Answer from the drawing. Dimensions are ordinates in mm from the lowest x, y and z of the part. A direction names the side the tool comes from. Round coordinates to 2 decimals unless told otherwise and drop trailing zeros. Loops run counter-clockwise (first coordinate to the right, second up) from the corner with the lowest first, then second, coordinate; pieces in that order, holes last. Notation, with made-up numbers: M -10.75,47 L 22.25,47 A21 ccw 22.25,57 Z; hole C 24.5,5.25 d10. An arc over 180 degrees is marked long. Answer as a JSON object with one key per item and string values.
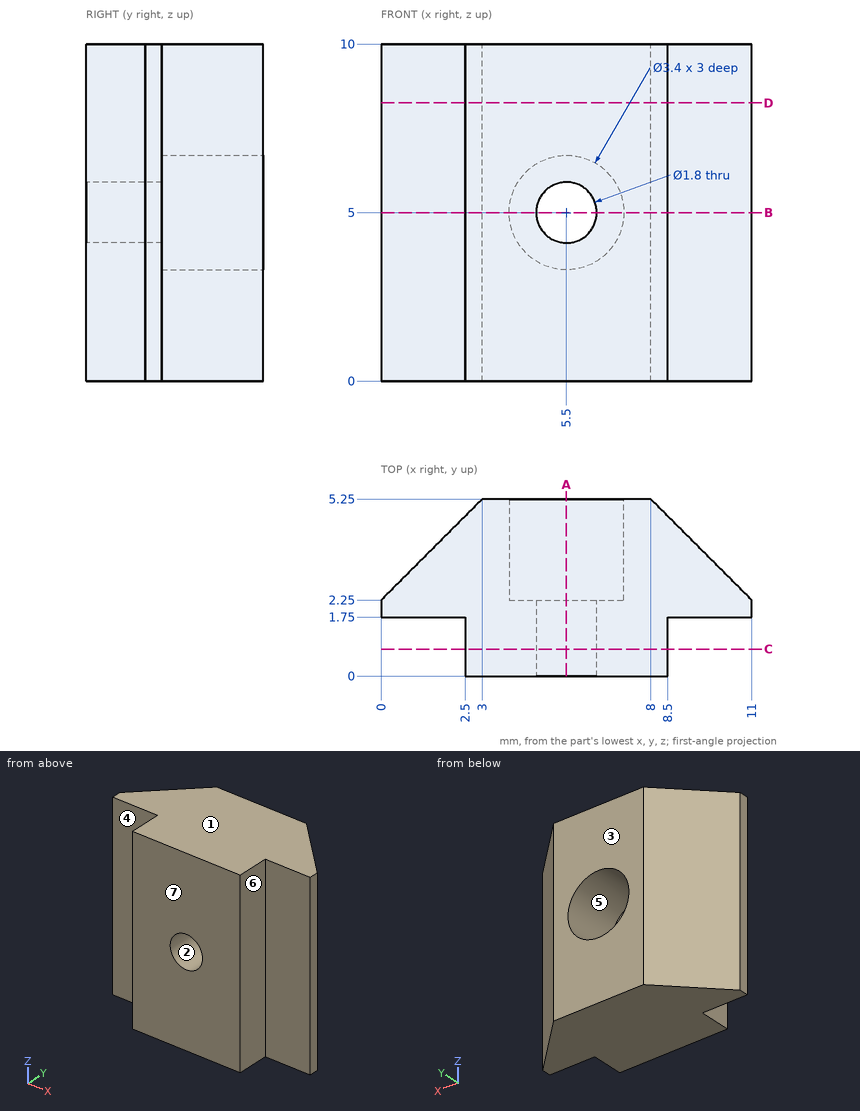
Item 1: The part is cut by section B-B (z = 5). Give the vertices of the cut face in (x, y).
Values follow:
{"outline": "M 0,1.75 L 2.5,1.75 L 2.5,0 L 4.6,0 L 4.6,2.25 L 3.8,2.25 L 3.8,5.25 L 3,5.25 L 0,2.25 Z; M 6.4,0 L 8.5,0 L 8.5,1.75 L 11,1.75 L 11,2.25 L 8,5.25 L 7.2,5.25 L 7.2,2.25 L 6.4,2.25 Z"}
Item 2: Straight lines are drawn through the part: line 1 (Z direction, x = 5.5, y = 0.45); line 2 (X direction, y = 1.6, z = 1); line 3 (X direction, y = 3.6, z = 4.5). For each, find the intervals that lie inside material, in ascending order.
Values follow:
{"line 1": "0 to 4.1, 5.9 to 10", "line 2": "2.5 to 8.5", "line 3": "1.35 to 3.88, 7.12 to 9.65"}
Item 3: Flat-ended cylindrical pins translate along their axes: P1, Ø1.4, axis at y = 0.5, z = 4.5, coming from the -X side; P2, Ø2, axis at x = 10.5, z = 3, coming from the -Y side; P3, Ø1.1, axis at x = 5.5, z = 5, coming from the -Y side; P4, Ø1, axis at y = 3, z = 6, coming from the -X side. Find the tip coordinate at first contact, or state that the pin passes through.
Values follow:
{"P1": "x = 2.5", "P2": "y = 1.75", "P3": "through", "P4": "x = 0.25"}
Item 4: Determine the mould class of the marked faces 1, 2 and 3 for opening direction Z: released by +Z, released by -Z, zero draft, split by the parting line, or undercut.
Values follow:
{"face 1": "released by +Z", "face 2": "undercut", "face 3": "zero draft"}
Item 5: The part is cut by section A-A (x = 5.5). Give the vertices of the cut face in (y, z).
Values follow:
{"outline": "M 0,0 L 5.25,0 L 5.25,3.3 L 2.25,3.3 L 2.25,4.1 L 0,4.1 Z; M 0,5.9 L 2.25,5.9 L 2.25,6.7 L 5.25,6.7 L 5.25,10 L 0,10 Z"}
Item 6: Which of the six approach directions +Z, -Z, +X, -X, +Y, -Y give full straight-line access (tool end or side, diameter ignored) to the marked faces 4, 5, 6 and 7?
Values follow:
{"face 4": "+Z, -Z, -X, -Y", "face 5": "+Y", "face 6": "+Z, -Z, +X, -Y", "face 7": "+Z, -Z, +X, -X, -Y"}
Item 7: The part is cut by section D-D (z = 8.25). Give the vertices of the cut face in (x, y), then the cut area to 3 significant figures.
Values follow:
{"outline": "M 0,1.75 L 2.5,1.75 L 2.5,0 L 8.5,0 L 8.5,1.75 L 11,1.75 L 11,2.25 L 8,5.25 L 3,5.25 L 0,2.25 Z", "area": "40.0 mm^2"}
Item 8: The part is cut by section C-C (y = 0.8). Give the vertices of the cut face in (x, z).
Values follow:
{"outline": "M 2.5,0 L 8.5,0 L 8.5,10 L 2.5,10 Z; hole C 5.5,5 d1.8"}
